Here's how the part is built. I have some questions about the finished solid (model axes, mm). Face numbers are marked on the shaded views. A direction names the side the tool comes from. Round coordinates to 2 decimals unless told otherwise and drop trailing zeros. Loops run counter-clockwise (first coordinate to the right, second up) from the corner with the lowest first, then second, coordinate; pieces in that order, holes last. Notation, with made-up numbers: (71.25, 6.25) - (85.25, 6.25) arc R20 ccw to (85.25, 38.25) - close; hole circle Ø8 at (-22.75, 60). An arc over 180 degrees is marked (long way). Return JSON: item names as keys, results as strings. Group by question number.
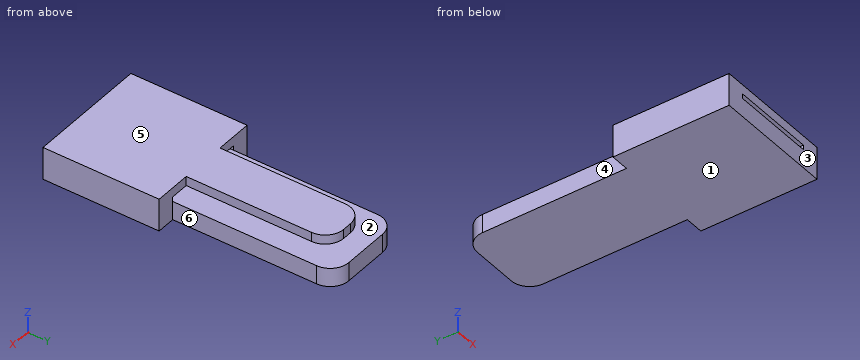
```python
from build123d import *

# Parameters (mm, degrees)
F0_W     = 2
F0_H     = 10
F0_W_2   = 9
F0_H_2   = 2.5
F0_H_3   = 15
F1_DEPTH = 2
F2_DEPTH = 0.5
F3_W     = 2
F3_H     = 10
F3_W_2   = 5
F3_H_2   = 15.5
F4_DEPTH = 1
F5_R     = 2
F6_DEPTH = 25
F7_DEPTH = 2.5


# Not quite as in the source:
# - a feature names something its author has since deleted; it is built from what else it names


with BuildPart() as f1:
    # F0 (on Top) → F1 (new body)
    with BuildSketch(Plane.XY):
        with Locations((-5.5, -7.5)):
            Rectangle(F0_W, F0_H)
        with Locations((0, 13.75)):
            Rectangle(F0_W_2, F0_H_2)
        Polygon((4.5, -2.5), (4.5, 12.5), (-4.5, 12.5), (-4.5, -2.5), (-4.5, -12.5), (4.5, -12.5), align=None)
        with Locations((0, -13.75)):
            Rectangle(F0_W_2, F0_H_2)
        with Locations((5.5, -7.5)):
            Rectangle(F0_W, F0_H)
        with Locations((-5.5, 5)):
            Rectangle(F0_W, F0_H_3)
        with Locations((5.5, 5)):
            Rectangle(F0_W, F0_H_3)
    extrude(amount=-F1_DEPTH)

    # F0 (on Top) → F2 (join)
    with BuildSketch(Plane.XY):
        with Locations((-5.5, -7.5)):
            Rectangle(F0_W, F0_H)
        with Locations((5.5, -7.5)):
            Rectangle(F0_W, F0_H)
    extrude(amount=F2_DEPTH)

    # F3 (on face) → F4 (join)
    with BuildSketch(Plane.XY.offset(0.5)):
        with Locations((-5.5, -7.5)):
            Rectangle(F3_W, F3_H)
        Polygon((-4.5, -2.5), (-4.5, -12.5), (6.5, -12.5), (6.5, -2.5), (4.5, -2.5), (2.5, -2.5), (-2.5, -2.5), align=None)
        with Locations((0, 5.25)):
            Rectangle(F3_W_2, F3_H_2)
    extrude(amount=F4_DEPTH)

    # F5
    f5_edges = [f1.edges().sort_by_distance(p)[0] for p in [
        (-4.5, 15, -1),
        (4.5, 15, -1),
        (-2.5, 13, 1),
        (2.5, 13, 1),
    ]]
    fillet(f5_edges, radius=F5_R)

    # F0 (on Top) → F6 (cut)
    with BuildSketch(Plane.XY):
        with Locations((-5.5, 5)):
            Rectangle(F0_W, F0_H_3)
        with Locations((5.5, 5)):
            Rectangle(F0_W, F0_H_3)
    extrude(amount=-F6_DEPTH, mode=Mode.SUBTRACT)

    # F7 (add, through all): a face of the model
    f7_faces = [f1.faces().sort_by_distance(p)[0] for p in [
        (-5.5, -12.5, -1.8653708798),
    ]]
    extrude(f7_faces, amount=F7_DEPTH)


solid = f1.part
```
Q1. Imagine slicing it at B-B, the plane x = -3.5. List the corners of the cut face in (y, z) for me, and give its area (3 significant figures).
Q2. Imagine slicing it at C-C, the plane z = -0.5. List the corners of the cut face in (x, y) for me.
Q3. If we mould it in two halves opening along Z, with no side actions, what happens to the marked faces 1, 2 and 3? For each: +Z half, -Z half, draft (parallel to the pull), parting line (faces both ways), or undercut.
Q4. Imagine slicing it at D-D, the plane y = -5.25. List the corners of the cut face in (x, z) for me, and give its area (3 significant figures).
Q5. For the marked faces 4, 5 and 6, which set-ups out of +Z, -Z, +X, -X, +Y, -Y let a thin tool reach every point of the face, with its end or its side?
Q6. Imagine slicing it at A-A, the plane y = 7.25. List the corners of the cut face in (x, z) for me, and give its area (3 significant figures).
Q7. Please list where these lines run through material, in increasing order: line 1 (X direction, y = -6.75, z = 0.45); line 2 (Z direction, x = 2, y = -5); line 3 (X direction, y = 10, z = -0.8).
Q8. Will these pins go through, and if not, where does the flat tip stop? pin 1 Ø1 at (y, z) = (8, -1.5) entering from -X; pin 2 Ø1 at (y, z) = (3, -1.5) entering from +X; pin 3 Ø0.8 at (y, z) = (3, 1) entering from -X.
Output values:
{
 "1": {"outline": "(-15, -2) - (14.73, -2) - (14.73, 0) - (-15, 0) - close; (-15, 0.5) - (-2.5, 0.5) - (-2.5, 1.5) - (-15, 1.5) - close", "area": "72.0 mm^2"},
 "2": {"outline": "(-6.5, -15) - (6.5, -15) - (6.5, -2.5) - (4.5, -2.5) - (4.5, 13) arc R2 ccw to (2.5, 15) - (-2.5, 15) arc R2 ccw to (-4.5, 13) - (-4.5, -2.5) - (-6.5, -2.5) - close"},
 "3": {"face 1": "-Z half", "face 2": "undercut", "face 3": "draft"},
 "4": {"outline": "(-6.5, -2) - (6.5, -2) - (6.5, 1.5) - (-6.5, 1.5) - close; hole (-4.5, 0) - (4.5, 0) - (4.5, 0.5) - (-4.5, 0.5) - close", "area": "41.0 mm^2"},
 "5": {"face 4": "+Z, -Z, -X, +Y", "face 5": "+Z, +X, -X, +Y, -Y", "face 6": "+Z, -Z, +X, +Y"},
 "6": {"outline": "(-4.5, -2) - (4.5, -2) - (4.5, 0) - (-4.5, 0) - close; (-2.5, 0.5) - (2.5, 0.5) - (2.5, 1.5) - (-2.5, 1.5) - close", "area": "23.0 mm^2"},
 "7": {"line 1": "x = -6.5 to -4.5, 4.5 to 6.5", "line 2": "z = -2 to 0, 0.5 to 1.5", "line 3": "x = -4.5 to 4.5"},
 "8": {"pin 1": "stops at x = -4.5", "pin 2": "stops at x = 4.5", "pin 3": "stops at x = -2.5"}
}
